from build123d import *

# Parameters (mm, degrees)
SALIENTE_EXTRUIR1_DEPTH           = 21
REDONDEO1_R                       = 1
RANURAS_DE_ESPIGA_DE_3_0MM1_D     = 3
RANURAS_DE_ESPIGA_DE_3_0MM1_DEPTH = 15
RANURAS_DE_ESPIGA_DE_3_0MM1_TIP   = 0.901290929


with BuildPart() as part:
    # Croquis1 → Saliente-Extruir1 (new body)
    with BuildSketch(Plane(origin=(0, 0, 0), x_dir=(1, 0, 0), z_dir=(0, 1, 0))):
        Polygon((-45.555555556, 0), (-45.555555556, 28.148148148), (101.481481481, 28.148148148), (101.481481481, 0), (91.481481481, 0), (91.481481481, 19.62962963), (-35.555555556, 19.62962963), (-35.555555556, 0), align=None)
    extrude(amount=SALIENTE_EXTRUIR1_DEPTH)

    # Redondeo1
    redondeo1_edges = [part.edges().sort_by_distance(p)[0] for p in [
        (27.962962963, 21, -19.62962963),
        (-35.555555556, 0, -9.814814815),
        (-40.555555556, 0, 0),
        (91.481481481, 21, -9.814814815),
        (-45.555555556, 10.5, -28.148148148),
        (101.481481481, 10.5, -28.148148148),
        (91.481481481, 10.5, -19.62962963),
        (96.481481481, 21, 0),
        (101.481481481, 21, -14.074074074),
        (27.962962963, 21, -28.148148148),
        (-45.555555556, 21, -14.074074074),
        (-40.555555556, 21, 0),
        (-35.555555556, 21, -9.814814815),
        (-45.555555556, 0, -14.074074074),
        (27.962962963, 0, -28.148148148),
        (101.481481481, 0, -14.074074074),
        (96.481481481, 0, 0),
        (91.481481481, 0, -9.814814815),
        (27.962962963, 0, -19.62962963),
    ]]
    fillet(redondeo1_edges, radius=REDONDEO1_R)

    # Ranuras de espiga de Ø3.0mm1
    with Locations(Plane.XY):
        with Locations((-41.007352785, 10.144878608), (96.462672376, 10.144878608)):
            Hole(RANURAS_DE_ESPIGA_DE_3_0MM1_D / 2, depth=RANURAS_DE_ESPIGA_DE_3_0MM1_DEPTH)
            with Locations((0, 0, -(RANURAS_DE_ESPIGA_DE_3_0MM1_DEPTH + RANURAS_DE_ESPIGA_DE_3_0MM1_TIP / 2))):  # 118° drill point
                Cone(0, RANURAS_DE_ESPIGA_DE_3_0MM1_D / 2, RANURAS_DE_ESPIGA_DE_3_0MM1_TIP, mode=Mode.SUBTRACT)


solid = part.part
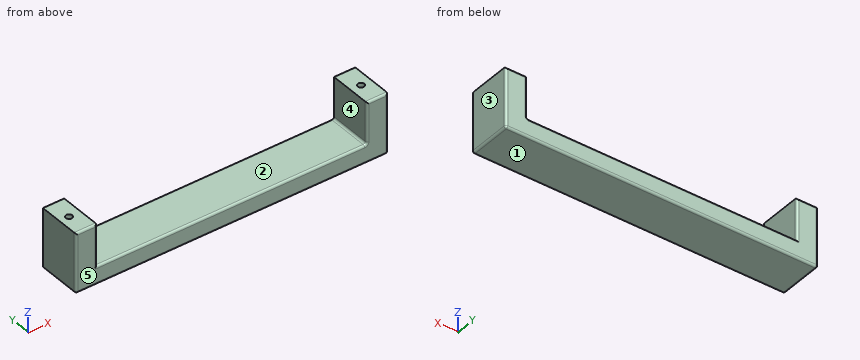
Can you work these out from the model? Positions are in its coordinate system, mm. Face numbers are marked on the shaded views. A direction names the side the tool comes from. Coordinates: 2 decimals unless noted, no trailing zeros. Order: outer loops, then holes, each group sorted by start corner. A loop starts at its lowest first (then second) coordinate and runs counter-clockwise, first axis right, second up. Notation, with made-up numbers: (15.25, 10.25) - (30.25, 10.25) arc R20 ccw to (30.25, 34.25) - close; hole circle Ø11 at (3, 40.5). An arc over 180 degrees is marked (long way). Answer as a JSON object with one key per item and string values. Group by question number.
Q1. I need wall thicknesses on line 1 (X direction, y = 19, z = -4.75); line 2 (X direction, y = 9, z = -11.5); line 3 (Z direction, x = 15, y = 12.25). Which ranges of each line are inside material? Lowest first, please. Write a range as from..to.
Q2. Imagine slicing it at A-A (z = -17.25). Please give me the cut outline in (x, y), and give its area (3 significant figures).
Q3. Imagine slicing it at C-C (x = 76.5). Please give me the cut outline in (y, z), and give its area (3 significant figures).
Q4. Will this pin go through, and if not, where does the flat tip stop? P1, Ø9.5, axis at x = 33.5, y = 13, coming from the +Z side.
Q5. On a 3-axis mill with a long thin cutter (end or side, diameter ignored), from which of +Z, -Z, +X, -X, +Y, -Y can I reach the whole of each face in a straight line? I mean the marked faces 4 and 5. Say none if no direction works.
Q6. We'd pull the mould along X, two halves only. Please class the marked faces 1, 2 and 3: +X half, -X half, draft (parallel to the pull), parting line (faces both ways), or undercut.
Q7. Imagine slicing it at B-B (y = 4). Please give me the cut outline in (x, z), and give its area (3 significant figures).
Determined:
{
 "1": {"line 1": "x = -45.56..-35.56, 91.48..101.48", "line 2": "x = -45.56..-41.98, -40.04..-35.56, 91.48..95.49, 97.43..101.48", "line 3": "z = -28.15..-19.63"},
 "2": {"outline": "(-45.56, 1) arc R1 ccw to (-44.56, 0) - (-36.56, 0) arc R1 ccw to (-35.56, 1) - (-35.56, 20) arc R1 ccw to (-36.56, 21) - (-44.56, 21) arc R1 ccw to (-45.56, 20) - close; (91.48, 1) arc R1 ccw to (92.48, 0) - (100.48, 0) arc R1 ccw to (101.48, 1) - (101.48, 20) arc R1 ccw to (100.48, 21) - (92.48, 21) arc R1 ccw to (91.48, 20) - close", "area": "418 mm2"},
 "3": {"outline": "(0, -27.15) arc R1 ccw to (1, -28.15) - (20, -28.15) arc R1 ccw to (21, -27.15) - (21, -20.63) arc R1 ccw to (20, -19.63) - (1, -19.63) arc R1 ccw to (0, -20.63) - close", "area": "178 mm2"},
 "4": {"P1": "stops at z = -19.63"},
 "5": {"face 4": "+Z, +Y, -Y", "face 5": "+Z, -Z, +X, -X, -Y"},
 "6": {"face 1": "draft", "face 2": "undercut", "face 3": "+X half"},
 "7": {"outline": "(-45.56, -27.15) arc R1 ccw to (-44.56, -28.15) - (100.48, -28.15) arc R1 ccw to (101.48, -27.15) - (101.48, 0) - (91.48, 0) - (91.48, -18.63) arc R1 cw to (90.48, -19.63) - (-35.56, -19.63) - (-35.56, 0) - (-45.56, 0) - close", "area": "1,640 mm2"}
}
